```python
from build123d import *

# Parameters (mm, degrees)
SKETCH1_R           = 39
BOSS_EXTRUDE1_DEPTH = 3.85
SKETCH2_R           = 2.5
SKETCH4_R           = 8
BOSS_EXTRUDE2_DEPTH = 8.9
SKETCH5_R           = 3.1
CUT_EXTRUDE1_DEPTH  = 15.6
SKETCH6_R           = 2
CUT_EXTRUDE2_DEPTH  = 57.608855314
SKETCH3_R           = 2.561236926


with BuildPart() as part:
    # Sketch1 → Boss-Extrude1 (new, symmetric)
    with BuildSketch(Plane.XY):
        with Locations(Location((0, 0, 0), (0, 0, 180))):
            Circle(SKETCH1_R)
    extrude(amount=BOSS_EXTRUDE1_DEPTH, both=True)

    # Cut-Sweep1: sweep along a curve in space
    with BuildLine() as cut_sweep1_path:
        ThreePointArc((39, 0, -3.85), (27.577164466, 27.577164466, -3.85), (0, 39, -3.85))
        ThreePointArc((0, 39, -3.85), (-27.577164466, 27.577164466, -3.85), (-39, 0, -3.85))
        ThreePointArc((-39, 0, -3.85), (-27.577164466, -27.577164466, -3.85), (0, -39, -3.85))
        ThreePointArc((0, -39, -3.85), (27.577164466, -27.577164466, -3.85), (39, 0, -3.85))
    # Sketch2 → Cut-Sweep1 (sweep, cut)
    with BuildSketch(Plane(origin=(0, 0, 0), x_dir=(1, 0, 0), z_dir=(0, 1, 0))):
        with Locations((39, 0)):
            Circle(SKETCH2_R)
    sweep(path=cut_sweep1_path.line, mode=Mode.SUBTRACT)

    # Sketch4 → Boss-Extrude2 (add)
    with BuildSketch(Plane.XY.offset(3.85)):
        Circle(SKETCH4_R)
    extrude(amount=BOSS_EXTRUDE2_DEPTH)

    # Sketch5 → Cut-Extrude1 (cut)
    with BuildSketch(Plane.XY.offset(12.75)):
        Circle(SKETCH5_R)
    extrude(amount=-CUT_EXTRUDE1_DEPTH, mode=Mode.SUBTRACT)

    # Sketch6 → Cut-Extrude2 (cut, through all)
    with BuildSketch(Plane(origin=(0, 0, 0), x_dir=(1, 0, 0), z_dir=(0, 1, 0))):
        with Locations(Location((0, -7.5, 0), (0, 0, 270))):
            Circle(SKETCH6_R)
    extrude(amount=-CUT_EXTRUDE2_DEPTH, mode=Mode.SUBTRACT)

    # Sketch3 → Revolve1 (revolve)
    with BuildSketch(Plane(origin=(0, 0, 0), x_dir=(1, 0, 0), z_dir=(0, 1, 0)), mode=Mode.PRIVATE) as revolve1_sk:
        with Locations((39, 0)):
            Circle(SKETCH3_R)
    revolve(revolve1_sk.sketch.rotate(Axis((0, 0, 12.75), (0, 0, -1)), 180), axis=Axis((0, 0, 12.75), (0, 0, -1)))


solid = part.part
```
CAD build for the part. Positions are in the model's coordinates, mm. A direction names the side the tool comes from. Round coordinates to 2 decimals unless told otherwise and drop trailing zeros. Write each loop counter-clockwise with the first axis right and the second up, starting at its lowest first coordinate (ties: lowest second). Pieces come first, ordered by that corner, then holes. Notation, with made-up numbers: (-27, 42.5) - (-7, 42.5) arc R14 ccw to (-7, 63.5) - close; hole circle Ø5 at (18.25, -28). An arc over 180 degrees is marked (long way). Return JSON: item names as keys, results as strings. Group by question number.
Item 1: Flat gauge pins, fed straight in: pin 1 Ø2 at (x, y) = (17, 2.5) entering from +Z; pin 2 Ø1 at (x, z) = (11, 1.5) entering from -Y; pin 3 Ø5 at (x, y) = (0, 0) entering from +Z. Where does each tip first touch, or does it go through?
Item 2: Band-saw the part on C-C on z = 7.5. List the corners of the cut face in (x, y).
Item 3: Mould opens along X. For faces 1 (the face through (4.301, 6.746, 8.238)), 2 (the face through (1, -9, 3.85)), 3 (the face through (-0.766, -5.148, 9.347)) say: +X half, -X half, draft (parallel to the pull), parting line (faces both ways), or undercut.
Item 4: 3-axis set-ups, long thin cutter, end or side, ignore diameter. For faces 4 (the face through (3.4, 0.1, 12.75)), 5 (the face through (5.077, -38.668, 3.215)), 6 (the face through (5.077, -38.668, -3.197)): which of +Z, -Z, +X, -X, +Y, -Y reach the whole face in a straight line?
Item 5: Probe probe 1 along Z at (x, y) = (0, -5.4); probe 2 along Z at (x, y) = (-37, -6.5); probe 3 along Z at (x, y) = (-34, -19.5). List the from-to ranges inside material, lowest first.
Item 6: Band-saw the part on A-A on x = 0. List the corners of the cut face in (y, z), plus the area to 3 significant figures.
Item 7: Band-saw the part on B-B on y = 0. List the corners of the cut face in (x, z).
Resolved:
{
 "1": {"pin 1": "stops at z = 3.85", "pin 2": "stops at y = -39.91", "pin 3": "stops at z = -2.85"},
 "2": {"outline": "(-2, -7.75) - (-2, -2.37) arc R3.1 cw (long way) to (2, -2.37) - (2, -7.75) arc R8 ccw (long way) to start"},
 "3": {"face 1": "parting line", "face 2": "draft", "face 3": "undercut"},
 "4": {"face 4": "+Z, +X, -X, +Y, -Y", "face 5": "+Z", "face 6": "-Z"},
 "5": {"probe 1": "z = -3.85 to 5.5, 9.5 to 12.75", "probe 2": "z = -3.85 to 3.85", "probe 3": "z = -2.55 to 2.55"},
 "6": {"outline": "(-39, -3.85) - (39, -3.85) - (39, -2.56) arc R2.56 ccw to (39, 2.56) - (39, 3.85) - (8, 3.85) - (8, 12.75) - (3.1, 12.75) - (3.1, -2.85) - (-3.1, -2.85) - (-3.1, 5.5) - (-8, 5.5) - (-8, 3.85) - (-39, 3.85) - (-39, 2.56) arc R2.56 ccw to (-39, -2.56) - close; (-8, 9.5) - (-3.1, 9.5) - (-3.1, 12.75) - (-8, 12.75) - close", "area": "647 mm²"},
 "7": {"outline": "(-39, -3.85) - (39, -3.85) - (39, -2.56) arc R2.56 ccw to (39, 2.56) - (39, 3.85) - (8, 3.85) - (8, 12.75) - (3.1, 12.75) - (3.1, -2.85) - (-3.1, -2.85) - (-3.1, 12.75) - (-8, 12.75) - (-8, 3.85) - (-39, 3.85) - (-39, 2.56) arc R2.56 ccw to (-39, -2.56) - close"}
}
